Source: CAD feature listing. Evaluate the final solid. Frame: model axes, mm. A direction names the side the tool comes from. Give positions to 0.01 mm unless a question says otherwise; leave off trailing zeros. Loops run counter-clockwise (first coordinate to the right, second up) from the corner with the lowest first, then second, coordinate; pieces in that order, holes last. Notation, with made-up numbers: M 49,-12 L 84,-12 A9 ccw 84,-4 Z; hole C -39.5,49 d4. An arc over 180 degrees is marked long. Put each result on its own line as item: value.
from build123d import *

# Parameters (mm, degrees)
F1_DEPTH = 9.525
F2_R     = 6.35
F2_R_2   = 3.2385
F3_DEPTH = 25.4
F5_DEPTH = 25.4


with BuildPart() as f1:
    # F0 (on Top) → F1 (new body)
    with BuildSketch(Plane.XY):
        with BuildLine():
            ThreePointArc((0, -30.988), (-8.980256, -34.707744), (-12.7, -43.688))
            ThreePointArc((-12.7, -43.688), (0, -56.388), (12.7, -43.688))
            ThreePointArc((12.7, -43.688), (8.980256, -34.707744), (0, -30.988))
        make_face()
        with BuildLine():
            ThreePointArc((0, 30.988), (-8.980256, 34.707744), (-12.7, 43.688))
            Line((-12.7, 43.688), (-12.7, -43.688))
            ThreePointArc((-12.7, -43.688), (-8.980256, -34.707744), (0, -30.988))
            Line((0, -30.988), (0, 30.988))
        make_face()
        with BuildLine():
            ThreePointArc((0, 30.988), (8.980256, 34.707744), (12.7, 43.688))
            ThreePointArc((12.7, 43.688), (0, 56.388), (-12.7, 43.688))
            ThreePointArc((-12.7, 43.688), (-8.980256, 34.707744), (0, 30.988))
        make_face()
    extrude(amount=F1_DEPTH)

    # F2 (on face) → F3 (cut)
    with BuildSketch(Plane.XY.offset(9.525)):
        with Locations((0, -43.688)):
            Circle(F2_R)
        with Locations((0, 43.688)):
            Circle(F2_R_2)
    extrude(amount=-F3_DEPTH, mode=Mode.SUBTRACT)

    # F4 (on Front) → F5 (join, symmetric)
    with BuildSketch(Plane.XZ):
        Polygon((0, 19.05), (-12.7, 19.05), (-12.7, 9.525), (-6.35, 9.525), (-6.35, 15.875), (-2.54, 15.875), (-2.54, 9.525), (0, 9.525), align=None)
    extrude(amount=F5_DEPTH, both=True)


solid = f1.part
1. Material intervals for line 1 (X direction, y = -19, z = 13.25); line 2 (Y direction, x = -2, z = 7); line 3 (Y direction, x = 1, z = 1.25), sorted ascending. Write a range as from..to.
Found:
line 1: -12.7..-6.35, -2.54..0
line 2: -56.23..-49.71, -37.66..41.14, 46.24..56.23
line 3: -56.35..-49.96, -37.42..-31.03, 31.03..40.61, 46.77..56.35
2. Section query C-C (z = 6.5). Output: boundary loops of the cut face in (x, y).
Found:
outline: M -12.7,-43.69 A12.7 ccw long 0,-30.99 L 0,30.99 A12.7 ccw long -12.7,43.69 Z; hole C 0,-43.69 d12.7; hole C 0,43.69 d6.48
3. Section query D-D (x = 10). Output: boundary loops of the cut face in (y, z) (3 decimals).
Found:
outline: M -51.517,0 L -35.859,0 L -35.859,9.525 L -51.517,9.525 Z; M 35.859,0 L 51.517,0 L 51.517,9.525 L 35.859,9.525 Z
4. Draft query along Z for faces 5 (the flat face through (-2.54, 0, 13)), 6 (the flat face through (-12.7, 1, 7)), 7 (the flat face through (-6, 0, 19.05)), 8 (the flat face through (-4, 0, 15.875)). Return one class per face: pulls with the +Z half, pulls with the -Z half, needs draft (parallel to the pull), parting line crosses it, or undercut.
Found:
face 5: undercut
face 6: needs draft
face 7: pulls with the +Z half
face 8: undercut
5. Access query for faces 1 (the flat face through (-6.35, 0, 13)), 2 (the flat face through (-8, -25.4, 14)), 3 (the flat face through (-8, 25.4, 14)), 4 (the flat face through (0, 0, 9)). Directions: +Z, -Z, +X, -X, +Y, -Y. A direction counts if a zero-diameter tool reaches every point of the face in a straight line with its end or side. Return the directions, or none.
Found:
face 1: +Y, -Y
face 2: +Z, +X, -X, -Y
face 3: +Z, +X, -X, +Y
face 4: +Z, -Z, +X
6. Contact query for flat-ended pins moving along their axis: P1, Ø5, axis at y = -9.5, z = 14, coming from the +X side; P2, Ø5, axis at x = -3, z = 14, coming from the -Y side; P3, Ø10.5, axis at x = -8, z = 12.5, coming from the +Y side. Output: stop coordinate, or through.
Found:
P1: x = 0
P2: y = -25.4
P3: y = 55.84
7. Section query B-B (y = -19.5). Output: boundary loops of the cut face in (x, z) (3 decimals).
Found:
outline: M -12.7,0 L 0,0 L 0,19.05 L -12.7,19.05 Z; hole M -6.35,9.525 L -2.54,9.525 L -2.54,15.875 L -6.35,15.875 Z
8. Section query A-A (z = 14). Output: boundary loops of the cut face in (x, y).
Found:
outline: M -12.7,-25.4 L -6.35,-25.4 L -6.35,25.4 L -12.7,25.4 Z; M -2.54,-25.4 L 0,-25.4 L 0,25.4 L -2.54,25.4 Z
